```python
from build123d import *

# Parameters (mm, degrees)
EXTRUDE_1_DEPTH          = 199
EXTRUDE_1_DEPTH_BACK     = 200
CUT_EXTRUDE_1_DEPTH      = 10
CUT_EXTRUDE_1_DEPTH_BACK = 30
SKETCH_3_R               = 9


with BuildPart() as part:
    # Эскиз1 → Вытянуть-Тонкостенный1 (new, two sides: drawn at the far end of the back side and taken through both)
    with BuildSketch(Plane(origin=(0, 0, 0), x_dir=(1, 0, 0), z_dir=(0, 1, 0)).offset(-EXTRUDE_1_DEPTH_BACK)):
        with BuildLine():
            Line((-6, 7.5), (6, 7.5))
            ThreePointArc((6, 7.5), (8.828427125, 6.328427125), (10, 3.5))
            Line((10, 3.5), (10, -3.5))
            ThreePointArc((10, -3.5), (8.828427125, -6.328427125), (6, -7.5))
            Line((6, -7.5), (-6, -7.5))
            ThreePointArc((-6, -7.5), (-8.828427125, -6.328427125), (-10, -3.5))
            Line((-10, -3.5), (-10, 3.5))
            ThreePointArc((-10, 3.5), (-8.828427125, 6.328427125), (-6, 7.5))
        make_face()
        with BuildLine():
            Line((-6, 5.5), (6, 5.5))
            ThreePointArc((6, 5.5), (7.414213562, 4.914213562), (8, 3.5))
            Line((8, 3.5), (8, -3.5))
            ThreePointArc((8, -3.5), (7.414213562, -4.914213562), (6, -5.5))
            Line((6, -5.5), (-6, -5.5))
            ThreePointArc((-6, -5.5), (-7.414213562, -4.914213562), (-8, -3.5))
            Line((-8, -3.5), (-8, 3.5))
            ThreePointArc((-8, 3.5), (-7.414213562, 4.914213562), (-6, 5.5))
        make_face(mode=Mode.SUBTRACT)
    extrude(amount=EXTRUDE_1_DEPTH + EXTRUDE_1_DEPTH_BACK)

    # Surface Cut 1
    split(bisect_by=Plane(origin=(49.080127019, 183.169527677, 0), x_dir=(0, 0, 1), z_dir=(0.25881904510252135, 0.9659258262890681, 0)), keep=Keep.BOTTOM)

    # Эскиз3 → Вырез-Вытянуть1 (cut, two sides: drawn at the far end of the back side and taken through both)
    with BuildSketch(Plane(origin=(-59.080127019, 15.830472323, 0), x_dir=(0, 0, 1), z_dir=(-0.9659258262890681, 0.25881904510252135, 0)).offset(-CUT_EXTRUDE_1_DEPTH_BACK)):
        with Locations((0, 194.63104898)):
            Circle(SKETCH_3_R)
    extrude(amount=CUT_EXTRUDE_1_DEPTH + CUT_EXTRUDE_1_DEPTH_BACK, mode=Mode.SUBTRACT)

    # Surface Cut 2
    split(bisect_by=Plane(origin=(-49.330127019, -184.102540378, 0), x_dir=(0, 0, -1), z_dir=(0.25881904510252135, 0.9659258262890681, 0)), keep=Keep.TOP)


solid = part.part
```
The listing builds one solid part. Answer for the finished solid, in the listing's coordinates (mm). A direction names the side the tool comes from. Round coordinates to 2 decimals unless told otherwise and drop trailing zeros. Order: outer loops, then holes, each group sorted by start corner. A loop starts at its lowest first (then second) coordinate and runs counter-clockwise, first axis right, second up. Notation, with made-up numbers: (32.5, 28) -> (39.5, 28) arc R28 cw to (39.5, 47) -> close; hole circle Ø4 at (16.25, 57). An arc over 180 degrees is marked (long way). Answer as CSV lines item,"result".
Q1. A cutting plane is placed at A-A on y = -121. Determine the outline of the cut face in (x, z).
Computed values:
outline,"(-10, -3.5) arc R4 ccw to (-6, -7.5) -> (6, -7.5) arc R4 ccw to (10, -3.5) -> (10, 3.5) arc R4 ccw to (6, 7.5) -> (-6, 7.5) arc R4 ccw to (-10, 3.5) -> close; hole (-8, -3.5) arc R2 ccw to (-6, -5.5) -> (6, -5.5) arc R2 ccw to (8, -3.5) -> (8, 3.5) arc R2 ccw to (6, 5.5) -> (-6, 5.5) arc R2 ccw to (-8, 3.5) -> close"
Q2. Consider line 1 (Z direction, x = -3, y = 97.5); line 2 (X direction, y = -93, z = -3.75); line 3 (X direction, y = -97, z = 4). Determine where each line is inside the solid, lowest interval first. Write a range as from..to.
Computed values:
line 1,"z = -7.5..-5.5, 5.5..7.5"
line 2,"x = -9.99..-7.98, 7.98..9.99"
line 3,"x = -9.97..-7.94, 7.94..9.97"
Q3. For a pull along Z with two mould halves and no side action, classify faces 3 (the flat face through (-10, -2, 0)), 4 (the flat face through (0, -3, -7.5)), 5 (the flat face through (8, -7, 0)), 6 (the flat face through (0, -3, 7.5)) as +Z half, -Z half, draft (parallel to the pull), parting line (faces both ways), or undercut.
Computed values:
face 3,"draft"
face 4,"-Z half"
face 5,"undercut"
face 6,"+Z half"
Q4. Which of the six approach directions +Z, -Z, +X, -X, +Y, -Y give full straight-line access (tool end or side, diameter ignored) to faces 1 (the flat face through (-8, -3, 0)), 2 (the flat face through (10, -8, 0))?
Computed values:
face 1,"+Y, -Y"
face 2,"+Z, -Z, +X, +Y, -Y"
Q5. A cutting plane is placed at B-B on z = 0.75. Determine the outline of the cut face in (x, y).
Computed values:
outline,"(-10, -194.64) -> (-8, -195.18) -> (-8, 194.36) -> (-10, 194.89) -> close; (8, -199.46) -> (10, -200) -> (10, 189.53) -> (8, 190.07) -> close"
Q6. Given pin 1 (2 mm diameter, centred on x = 7, z = -4.5, fed in from +Y), flat-ended and moving along its own axis, determine where the tip first touches the part or whether it passes through.
Computed values:
pin 1,"stops at y = 192.29"
